```python
from build123d import *

# Parameters (mm, degrees)
F1_DEPTH = 9
F3_W     = 20
F3_H     = 3.8
F4_DEPTH = 25
F6_D     = 3.3
F7_D     = 3.3
F8_R     = 3


with BuildPart() as f1:
    # F0 (on Top) → F1 (new body)
    with BuildSketch(Plane.XY):
        Polygon((8, 2), (-8, 2), (-8, -2), (0.259353, -2), (9.756975, -18.450364), (17.294511, -14.098566), align=None)
    extrude(amount=F1_DEPTH)

    # F3 (on face) → F4 (cut)
    with BuildSketch(Plane(origin=(6.866025, 3.964102, 0), x_dir=(-0.5, 0.866025, 0), z_dir=(0.866025, 0.5, 0))):
        with Locations((-20.856972, 4.5)):
            Rectangle(F3_W, F3_H)
    extrude(amount=-F4_DEPTH, mode=Mode.SUBTRACT)

    # F6 (through all)
    with Locations(Plane.XY.offset(9)):
        with Locations((11.525743, -12.810364)):
            Hole(F6_D / 2)

    # F7 (through all)
    with Locations(Plane(origin=(0, 2, 0), x_dir=(-1, 0, 0), z_dir=(0, 1, 0))):
        with Locations((4.2, 4.5)):
            Hole(F7_D / 2)

    # F8
    f8_edges = [f1.edges().sort_by_distance(p)[0] for p in [
        (-8, 0, 9),
        (-8, 0, 0),
        (8, 2, 4.5),
        (17.294511, -14.098566, 7.7),
        (17.294511, -14.098566, 1.3),
        (9.756975, -18.450364, 7.7),
        (9.756975, -18.450364, 1.3),
    ]]
    fillet(f8_edges, radius=F8_R)


solid = f1.part
```
Geometry: final body of the model. Coordinates: model frame, mm. A direction names the side the tool comes from. Give positions to 0.01 mm unless a question says otherwise; leave off trailing zeros. Loops run counter-clockwise (first coordinate to the right, second up) from the corner with the lowest first, then second, coordinate; pieces in that order, holes last. Notation, with made-up numbers: (28, 82) -> (84, 82) arc R26 ccw to (84, 107) -> close; hole circle Ø6 at (25, 41). An arc over 180 degrees is marked (long way). Return JSON: item names as keys, results as strings.
Item 1: Access query for faces 1 (the flat face through (-2, -2, 4)), 2 (the flat face through (11.61, -4.25, 4.44)), 3 (the flat face through (11, -11, 2.6)). Directions: +Z, -Z, +X, -X, +Y, -Y. A direction counts if a zero-diameter tool reaches every point of the face in a straight line with its end or side. Return the directions, or none.
Filled in:
{"face 1": "+Z, -Z, -X, -Y", "face 2": "+Z, -Z, +X, +Y", "face 3": "+X, -Y"}
Item 2: Mould query, pull axis Z, two halves, no side actions, for faces 4 (the flat face through (5, -5, 9)), 5 (the flat face through (5, -5, 0)), 6 (the flat face through (8.579, -7.584, 4.473)). Classes: released by +Z, released by -Z, zero draft, split by the parting line, or undercut.
Filled in:
{"face 4": "released by +Z", "face 5": "released by -Z", "face 6": "undercut"}
Item 3: Line query: line 1 (Z direction, x = -4.2, y = -0.45); line 2 (Y direction, x = 11.25, z = 7.75); line 3 (Y direction, x = -6, z = 2). Output: solid intervals per line, ascending.
Filled in:
{"line 1": "0 to 2.85, 6.15 to 9", "line 2": "-17.33 to -14.44, -11.18 to -3.63", "line 3": "-2 to 2"}
Item 4: Section C-C, the plane y = -12. Output: boundary loops of the cut face in (x, z), plus the area to 3 significant figures.
Filled in:
{"outline": "(6.03, 0) -> (10.09, 0) -> (10.09, 2.6) -> (6.03, 2.6) -> close; (6.03, 6.4) -> (10.09, 6.4) -> (10.09, 9) -> (6.03, 9) -> close; (12.96, 0) -> (16.02, 0) -> (16.02, 2.6) -> (12.96, 2.6) -> close; (12.96, 6.4) -> (16.02, 6.4) -> (16.02, 9) -> (12.96, 9) -> close", "area": "37.0 mm^2"}
Item 5: Section A-A, the plane z = 4.5. Output: boundary loops of the cut face in (x, y).
Filled in:
{"outline": "(-8, -2) -> (-5.85, -2) -> (-5.85, 2) -> (-8, 2) -> close; (-2.55, -2) -> (0.26, -2) -> (4.76, -9.79) -> (12.29, -5.44) -> (8.87, 0.5) arc R3 ccw to (6.27, 2) -> (-2.55, 2) -> close"}
Item 6: Section D-D, the plane x = 12.75. Output: boundary loops of the cut face in (y, z).
Filled in:
{"outline": "(-16.72, 0) -> (-13.92, 0) -> (-13.92, 2.6) -> (-16.72, 2.6) -> close; (-16.72, 6.4) -> (-13.92, 6.4) -> (-13.92, 9) -> (-16.72, 9) -> close; (-11.7, 0) -> (-6.23, 0) -> (-6.23, 2.6) -> (-11.7, 2.6) -> close; (-11.7, 6.4) -> (-6.23, 6.4) -> (-6.23, 9) -> (-11.7, 9) -> close"}
Item 7: Section B-B, the plane x = -4.2. Output: boundary loops of the cut face in (y, z), plus the area to 3 significant figures.
Filled in:
{"outline": "(-2, 0) -> (2, 0) -> (2, 2.85) -> (-2, 2.85) -> close; (-2, 6.15) -> (2, 6.15) -> (2, 9) -> (-2, 9) -> close", "area": "22.8 mm^2"}
Item 8: Pin query (flat end, axial travel): P1, Ø3, axis at y = -12, z = 2.5, coming from the -X side; P2, Ø4, axis at x = 11.53, y = -12.81, coming from the +Z side; P3, Ø3, axis at y = -7.5, z = 1, coming from the +X side; P4, Ø1, axis at y = -14.5, z = 6.5, coming from the +X side. Return the tip coordinate at first contact, or that it passes through.
Filled in:
{"P1": "x = 5.17", "P2": "z = 9", "P3": "x = 14.35", "P4": "x = 16.03"}
